Autodesk Fusion 360 part; units mm, degrees
sketch "Sketch1" plane through (0, 0, 0) normal (0, 0, 1) x (1, 0, 0)
  line L0 (100, 50) -> (100, 20)
  line L1 (100, 50) -> (150, 50)
  line L2 (120, 20) -> (100, 20)
  line L3 (70, 50) -> (70, 70)
  line L4 (70, 70) -> (150, 70)
  line L5 (100, 50) -> (120, 50)
  line L6 (120, 50) -> (120, 20)
  line L7 (150, 50) -> (150, 70)
  line L8 (150, 50) -> (100, 50)
  line L9 (70, 50) -> (150, 50)
  line L10 (120, 50) -> (150, 50)
  line L11 (100, 50) -> (70, 50)
  line L12 (120, 50) -> (125, 50)
  line L13 (125, 20) -> (125, 50)
  line L14 (125, 20) -> (120, 20)
  line L15 (100, 20) -> (95, 20)
  line L16 (95, 20) -> (95, 50)
  dimension "d1" = 30
  dimension "d2" = 50
  dimension "d3" = 20
extrude "Extrude1" add sketch "Sketch1" along normal blind 60
sketch "Sketch2" plane through (0, 20, 0) normal (0, -1, 0) x (1, 0, 0)
  line L0 (95, 0) -> (125, 0)
  line L1 (125, 0) -> (125, 60)
  line L2 (125, 60) -> (95, 60)
  line L3 (95, 60) -> (95, 0)
  line L4 (95, 0) -> (100, 0)
  line L5 (100, 0) -> (100, 55)
  line L6 (100, 55) -> (120, 55)
  line L7 (120, 55) -> (120, 5)
  line L8 (120, 5) -> (100, 5)
  line L9 (-15, -85) -> (-10, -80)
  dimension "d6" = 5
extrude "Extrude2" add 1 faces at (105, 63.3333, 60) along direction (0, 0, 1) blind 2
extrude "Extrude3" cut sketch "Sketch2" against normal blind 30 contours L5 L6 L7 L8
extrude "Extrude4" cut 1 faces at (106.6667, 30, 55) along direction (0, 0, 1) blind 2
extrude "Extrude5" add 1 faces at (125, 40, 41.3333) along direction (1, 0, 0) blind 2
extrude "Extrude6" cut 1 faces at (120, 30, 39.6667) along direction (1, 0, 0) blind 2
sketch "Sketch3" plane through (0, 70, 0) normal (0, 1, 0) x (-1, 0, 0)
  line L0 (-150, 0) -> (-70, 0)
  line L1 (-70, 0) -> (-70, 62)
  line L2 (-70, 62) -> (-150, 62)
  line L3 (-150, 62) -> (-150, 0)
  line L4 (-70, 31) -> (-150, 31)
  line L5 (-150, 31) -> (-150, 16)
  line L6 (-150, 31) -> (-150, 46)
  line L7 (-150, 16) -> (-70, 16)
  line L8 (-150, 46) -> (-70, 46)
  dimension "d17" = 15
  dimension "d18" = 15
extrude "Extrude7" cut sketch "Sketch3" against normal blind 16 contours L0 L1 L3 L7 | L1 L2 L3 L8
sketch "Sketch4" plane through (0, 0, 0) normal (0, 0, -1) x (1, 0, 0)
  line L0 (70, -54) -> (150, -54)
  line L1 (150, -54) -> (150, -50)
  line L2 (150, -50) -> (127, -50)
  line L3 (127, -50) -> (127, -20)
  line L4 (127, -20) -> (95, -20)
  line L5 (95, -20) -> (95, -50)
  line L6 (95, -50) -> (70, -50)
  line L7 (70, -50) -> (70, -54)
  line L8 (127, -50) -> (127, -54)
  line L9 (95, -50) -> (95, -54)
sketch "Sketch5" plane through (0, 54, 0) normal (0, 1, 0) x (-1, 0, 0)
  line L0 (-150, 0) -> (-70, 0)
  line L1 (-70, 0) -> (-70, 16)
  line L2 (-70, 16) -> (-150, 16)
  line L3 (-150, 16) -> (-150, 0)
  line L4 (-95, 0) -> (-95, 16)
  line L5 (-126.9826, 0) -> (-126.9826, 16)
extrude "Extrude8" cut sketch "Sketch5" against normal blind 50 contours L0 L2 L3 L5 | L0 L1 L2 L4
sketch "Sketch6" plane through (0, 0, 62) normal (0, 0, 1) x (-1, 0, 0)
  line L0 (-150, -54) -> (-70, -54)
  line L1 (-70, -54) -> (-70, -50)
  line L2 (-70, -50) -> (-95, -50)
  line L3 (-95, -50) -> (-95, -20)
  line L4 (-95, -20) -> (-127, -20)
  line L5 (-127, -20) -> (-127, -50)
  line L6 (-127, -50) -> (-150, -50)
  line L7 (-150, -50) -> (-150, -54)
  line L8 (-127, -50) -> (-127, -54)
  line L9 (-127, -54) -> (-95, -50)
  line L10 (-95, -54) -> (-95, -50)
sketch "Sketch7" plane through (0, 54, 0) normal (0, 1, 0) x (-1, 0, 0)
  line L0 (-150, 46) -> (-70, 46)
  line L1 (-70, 46) -> (-70, 62)
  line L2 (-70, 62) -> (-150, 62)
  line L3 (-150, 62) -> (-150, 46)
  line L4 (-95.1201, 62) -> (-95.1201, 46)
  line L5 (-127.0485, 62) -> (-127.0485, 46)
extrude "Extrude9" cut sketch "Sketch7" against normal blind 50 contours L0 L2 L3 L5 | L0 L1 L2 L4
sketch "Sketch8" plane through (0, 0, 0) normal (0, 0, -1) x (1, 0, 0)
extrude "Extrude10" add 1 faces at (96.6667, 70, 36) along direction (0, 1, 0) blind 9
sketch "Sketch9" plane through (0, 0, 62) normal (0, 0, 1) x (1, 0, 0)
sketch "Sketch10" plane through (70, 0, 0) normal (-1, 0, 0) x (0, -1, 0)
  line L0 (-50, 46) -> (-79, 46)
  line L1 (-79, 46) -> (-79, 16)
  line L2 (-79, 16) -> (-50, 16)
  line L3 (-50, 16) -> (-50, 46)
  line L4 (-74, 27.7711) -> (-74, 16)
  line L5 (-74, 27.7711) -> (-74, 46)
  line L6 (-74, 46) -> (-54, 46)
  line L7 (-54, 16) -> (-54, 46)
  line L8 (-54, 16) -> (-54, 21)
  line L9 (-54, 21) -> (-74, 21)
  line L10 (-74, 21) -> (-74, 41)
  line L11 (-74, 41) -> (-54, 41)
  dimension "d28" = 20
  dimension "d29" = 5
  dimension "d30" = 20
extrude "Extrude11" cut sketch "Sketch10" against normal blind 500 contours L4 L5 L7 L9 L10 L11
sketch "Sketch11" plane through (0, 0, 0) normal (0, 1, 0) x (1, 0, 0)
sketch "Sketch12" plane through (0, 79, 0) normal (0, 1, 0) x (-1, 0, 0)
  line L0 (-150, 16) -> (-70, 16)
  line L1 (-70, 16) -> (-70, 46)
  line L2 (-70, 46) -> (-150, 46)
  line L3 (-150, 46) -> (-150, 16)
  line L4 (-94.9405, 16) -> (-94.9405, 46)
  line L5 (-126.875, 16) -> (-126.875, 46)
  line L6 (-94.9405, 16) -> (-99.9405, 16)
  line L7 (-126.875, 16) -> (-121.875, 16)
  line L8 (-99.9405, 16) -> (-105, 16)
  line L9 (-121.875, 16) -> (-116.875, 16)
  line L10 (-105, 16) -> (-105, 46)
  line L11 (-116.875, 16) -> (-116.875, 46)
  dimension "d33" = 5
  dimension "d34" = 5
  dimension "d35" = 5
extrude "Extrude12" cut sketch "Sketch12" against normal blind 25 contours L0 L2 L10 L11
sketch "Sketch13" plane through (0, 79, 0) normal (0, 1, 0) x (-1, 0, 0)
  line L0 (-105, 46) -> (-105, 16)
  line L1 (-105, 16) -> (-70, 16)
  line L2 (-70, 16) -> (-70, 46)
  line L3 (-70, 46) -> (-105, 46)
  line L4 (-70, 16) -> (-75, 16)
  line L5 (-70, 16) -> (-70, 21)
  line L6 (-105, 46) -> (-105, 41)
  line L7 (-105, 46) -> (-100, 46)
  line L8 (-105, 16) -> (-105, 17)
  line L9 (-105, 16) -> (-105, 21)
  line L10 (-105, 16) -> (-100, 16)
  line L11 (-70, 46) -> (-75, 46)
  line L12 (-70, 46) -> (-70, 41)
  line L13 (-94, 41) -> (-81, 41)
  line L14 (-75, 25.1667) -> (-75, 36.8333)
  line L15 (-100, 25.1667) -> (-100, 36.8333)
  line L16 (-81, 21) -> (-94, 21)
  line L17 (-75, 36.8333) -> (-82, 31)
  line L18 (-87.5, 26.4167) -> (-94, 21)
  line L19 (-81, 41) -> (-87.5, 35.5833)
  line L20 (-93, 31) -> (-100, 25.1667)
  line L21 (-100, 36.8333) -> (-93, 31)
  line L22 (-87.5, 26.4167) -> (-81, 21)
  line L23 (-75, 25.1667) -> (-82, 31)
  line L24 (-87.5, 35.5833) -> (-94, 41)
  dimension "d38" = 5
  dimension "d39" = 5
  dimension "d40" = 5
  dimension "d41" = 5
  dimension "d42" = 5
  dimension "d43" = 5
  dimension "d44" = 5
extrude "Extrude13" cut sketch "Sketch13" against normal blind 5 contours L13 L19 L24 | L14 L17 L23 | L15 L20 L21 | L16 L18 L22
sketch "Sketch14" plane through (0, 79, 0) normal (0, 1, 0) x (-1, 0, 0)
  line L0 (-116.875, 16) -> (-116.875, 46)
  line L1 (-116.875, 46) -> (-150, 46)
  line L2 (-150, 46) -> (-150, 16)
  line L3 (-150, 16) -> (-116.875, 16)
sketch "Sketch15" plane through (0, 0, 46) normal (0, 0, 1) x (-1, 0, 0)
  line L0 (-105, -54) -> (-105, -79)
  line L1 (-105, -79) -> (-70, -79)
  line L2 (-70, -79) -> (-70, -50)
  line L3 (-70, -50) -> (-95, -50)
  line L4 (-95, -50) -> (-95, -20)
  line L5 (-95, -20) -> (-95.1201, -20)
  line L6 (-95.1201, -20) -> (-95.1201, -54)
  line L7 (-95.1201, -54) -> (-105, -54)
  line L8 (-84.9539, -79) -> (-84.9539, -74)
  line L9 (-84.9539, -74) -> (-84.9539, -64)
  circle A0 centre (-84.9539, -64) radius 2.5
  dimension "d47" = 5
  dimension "d48" = 10
  dimension "d49" = 5
extrude "Extrude14" cut sketch "Sketch15" against normal blind 10 contours A0
sketch "Sketch16" plane through (0, 79, 0) normal (0, 1, 0) x (-1, 0, 0)
  line L0 (-81, 21) -> (-94, 21)
  line L1 (-94, 21) -> (-87.5, 26.4167)
  line L2 (-87.5, 26.4167) -> (-81, 21)
  line L3 (-75, 25.1667) -> (-82, 31)
  line L4 (-82, 31) -> (-75, 36.8333)
  line L5 (-75, 36.8333) -> (-75, 25.1667)
  line L6 (-93, 31) -> (-100, 25.1667)
  line L7 (-100, 25.1667) -> (-100, 36.8333)
  line L8 (-100, 36.8333) -> (-93, 31)
  line L9 (-94, 41) -> (-81, 41)
  line L10 (-81, 41) -> (-87.5, 35.5833)
  line L11 (-87.5, 35.5833) -> (-94, 41)
  line L12 (-105, 46) -> (-105, 16)
  line L13 (-105, 16) -> (-70, 16)
  line L14 (-70, 16) -> (-70, 46)
  line L15 (-70, 46) -> (-105, 46)
  line L16 (-117, 16) -> (-122, 16)
  line L17 (-117, 16) -> (-117, 21)
  line L18 (-117, 46) -> (-122, 46)
  line L19 (-117, 46) -> (-117, 41)
  line L20 (-150, 46) -> (-145, 46)
  line L21 (-150, 46) -> (-150, 41)
  line L22 (-150, 16) -> (-145, 16)
  line L23 (-150, 16) -> (-150, 21)
  line L24 (-150, 21) -> (-117, 21)
  line L25 (-122, 16) -> (-122, 46)
  line L26 (-117, 41) -> (-150, 41)
  line L27 (-145, 46) -> (-145, 16)
  dimension "d52" = 5
  dimension "d53" = 5
  dimension "d54" = 5
  dimension "d55" = 5
  dimension "d56" = 5
  dimension "d57" = 5
  dimension "d58" = 5
  dimension "d59" = 5
extrude "Extrude15" cut sketch "Sketch16" against normal blind 6 contours L24 L25 L26 L27
sketch "Sketch17" plane through (0, 0, 46) normal (0, 0, 1) x (-1, 0, 0)
  circle A0 centre (-84.9539, -64) radius 2.5
  line L0 (-105, -54) -> (-105, -79)
  line L1 (-105, -79) -> (-70, -79)
  line L2 (-70, -79) -> (-70, -50)
  line L3 (-70, -50) -> (-95, -50)
  line L4 (-95, -50) -> (-95, -20)
  line L5 (-95, -20) -> (-95.1201, -20)
  line L6 (-95.1201, -20) -> (-95.1201, -54)
  line L7 (-95.1201, -54) -> (-105, -54)
  line L8 (-117, -79) -> (-122, -79)
  line L9 (-117, -79) -> (-117, -74)
  line L10 (-150, -79) -> (-150, -74)
  line L11 (-150, -79) -> (-145, -79)
  line L12 (-150, -50) -> (-150, -55)
  line L13 (-150, -50) -> (-145, -50)
  line L14 (-145, -50) -> (-117, -50)
  line L15 (-117, -50) -> (-117, -55)
  line L16 (-117, -55) -> (-117, -50)
  line L17 (-117, -50) -> (-122, -50)
  line L18 (-122, -79) -> (-122, -50)
  line L19 (-117, -55) -> (-150, -55)
  line L20 (-145, -50) -> (-145, -79)
  line L21 (-150, -74) -> (-117, -74)
  dimension "d62" = 5
  dimension "d63" = 5
  dimension "d64" = 5
  dimension "d65" = 5
  dimension "d66" = 5
extrude "Extrude16" cut sketch "Sketch17" against normal blind 6 contours L18 L19 L20 L21
sketch "Sketch18" plane through (0, 0, 16) normal (0, 0, -1) x (1, 0, 0)
  line L0 (116.875, -54) -> (116.875, -79)
  line L1 (116.875, -79) -> (150, -79)
  line L2 (150, -79) -> (150, -50)
  line L3 (150, -50) -> (127, -50)
  line L4 (127, -50) -> (127, -20)
  line L5 (127, -20) -> (126.9826, -20)
  line L6 (126.9826, -20) -> (126.9826, -54)
  line L7 (126.9826, -54) -> (116.875, -54)
  line L8 (150, -79) -> (145, -79)
  line L9 (150, -79) -> (150, -75)
  line L10 (150, -50) -> (145, -50)
  line L11 (150, -50) -> (150, -55)
  line L12 (116.875, -79) -> (116.875, -74)
  line L13 (116.875, -79) -> (121.875, -79)
  line L14 (127, -50) -> (117, -50)
  line L15 (117, -50) -> (117, -58)
  line L16 (117, -58) -> (117, -50)
  line L17 (117, -50) -> (117, -55)
  line L18 (117, -50) -> (122, -50)
  line L19 (122, -50) -> (121.875, -79)
  line L20 (117, -55) -> (150, -55)
  line L21 (145, -50) -> (145, -79)
  line L22 (150, -75) -> (150, -74)
  line L23 (150, -74) -> (116.875, -74)
  dimension "d69" = 5
  dimension "d70" = 5
  dimension "d71" = 5
  dimension "d72" = 5
  dimension "d73" = 5
  dimension "d74" = 5
  dimension "d75" = 5
  dimension "d76" = 1
extrude "Extrude17" cut sketch "Sketch18" against normal blind 6 contours L19 L20 L21 L23
sketch "Sketch19" plane through (0, 0, 16) normal (0, 0, -1) x (1, 0, 0)
  line L0 (105, -79) -> (105, -54)
  line L1 (105, -54) -> (95, -54)
  line L2 (95, -54) -> (95, -50)
  line L3 (95, -50) -> (70, -50)
  line L4 (70, -50) -> (70, -79)
  line L5 (70, -79) -> (105, -79)
  line L6 (105, -79) -> (100, -79)
  line L7 (105, -79) -> (105, -74)
  line L8 (70, -79) -> (70, -74)
  line L9 (70, -79) -> (75, -79)
  line L10 (70, -50) -> (70, -55)
  line L11 (70, -50) -> (75, -50)
  line L12 (105, -54) -> (105, -50)
  line L13 (105, -50) -> (105, -55)
  line L14 (105, -50) -> (100, -50)
  line L15 (100, -50) -> (105, -50)
  line L16 (100, -79) -> (100, -50)
  line L17 (105, -55) -> (70, -55)
  line L18 (75, -50) -> (75, -79)
  line L19 (70, -74) -> (105, -74)
  dimension "d79" = 5
  dimension "d80" = 5
  dimension "d81" = 5
  dimension "d82" = 5
  dimension "d83" = 5
  dimension "d84" = 5
  dimension "d85" = 5
  dimension "d86" = 5
extrude "Extrude18" cut sketch "Sketch19" against normal blind 6 contours L16 L17 L18 L19
extrude "Extrude19" add 1 faces at (146.6667, 74, 34.3333) along direction (0, -1, 0) blind 20
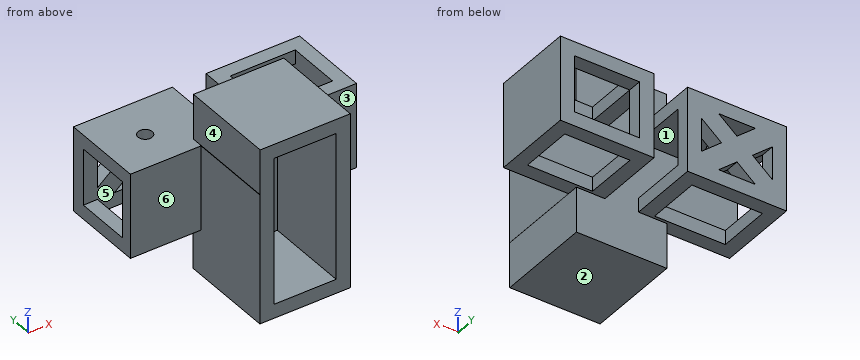
The listing builds one solid part. Answer for the finished solid, in the listing's coordinates (mm). Face numbers are marked on the shaded views. A direction names the side the tool comes from. Round coordinates to 2 decimals unless told otherwise and drop trailing zeros. Order: outer loops, then holes, each group sorted by start corner. A loop starts at its lowest first (then second) coordinate and runs counter-clockwise, first axis right, second up. Notation, with made-up numbers: (7, -31.5) - (18, -31.5) arc R24 ccw to (18, -2.5) - close; hole circle Ø2 at (57.5, -14.5). An arc over 180 degrees is marked (long way). Write item = value, one per line. Start each with the question number.
1) Section A-A, the plane x = 124.5 is taken. Write down the section's boundary in (y, z).
2) Section B-B, the plane z = 7.5 is taken. Write down the section's boundary in (x, y).
3) Given pin 1 (2 mm diameter, centred on x = 84.5, z = 41, fed in from -Y); pin 2 (8 mm diameter, centred on y = 42.5, z = 44.5, fed in from +X); pin 3 (4.5 mm diameter, centred on x = 84.95, y = 64, fed in from -Z); pin 4 (12.5 mm diameter, centred on x = 88.5, y = 62.5, fed in from -Z), each flat-ended and moving along its own axis, determine where each tip first touches the part or whether it passes through.
4) For the marked faces 4, 5 and 6, determine the directions among +Z, -Z, +X, -X, +Y, -Y from which every point of the face is accessible in a straight line to the end or side of a thin tool.
5) Straight lines are drawn through the part: L1, parallel to X at y = 64, z = 42.8 (3 decimals); L2, parallel to Z at x = 110, y = 34; L3, parallel to X at y = 37.5, z = 22.5. For each, find the intervals that lie inside material, in ascending order.
6) For a pull along Z with two mould halves and no side action, classify the marked faces 1, 2 and 3 as released by +Z, released by -Z, zero draft, split by the parting line, or undercut.
7) Section D-D, the plane z = 28.5 is taken. Count the separate pieces of the cut face and the enclosed holes in it, plus the area to 3 significant figures.
Results list:
q1.outline = (20, 0) - (54, 0) - (54, 16) - (55, 16) - (55, 21) - (54, 21) - (54, 41) - (55, 41) - (55, 46) - (54, 46) - (54, 62) - (20, 62) - close; (74, 16) - (79, 16) - (79, 21) - (74, 21) - close; (74, 41) - (79, 41) - (79, 46) - (74, 46) - close
q2.outline = (95, 20) - (100, 20) - (100, 50) - (122, 50) - (122, 20) - (126.98, 20) - (126.98, 54) - (95, 54) - close
q3.pin_1 = 50
q3.pin_2 = 127
q3.pin_3 = through
q3.pin_4 = 41
q4.face_4 = +Z, -X, +Y, -Y
q4.face_5 = none
q4.face_6 = +Z, -Z, -X, -Y
q5.L1 = 70 to 82.454, 87.454 to 105, 116.875 to 122, 145 to 150
q5.L2 = 0 to 5, 57 to 62
q5.L3 = 95 to 100, 122 to 127
q6.face_1 = undercut
q6.face_2 = released by -Z
q6.face_3 = zero draft
q7.separate_pieces = 5
q7.enclosed_holes = 0
q7.area = 906 mm^2
